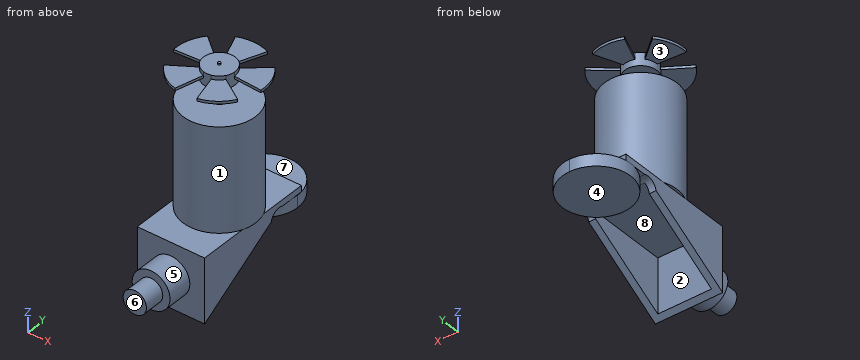
from build123d import *

# Parameters (mm, degrees)
F1_DEPTH  = 50.8
F2_R      = 3.175
F3_DEPTH  = 2.54
F4_R      = 0.635
F5_DEPTH  = 8.0518
F6_R      = 7.7597
F7_DEPTH  = 3.175
F9_DEPTH  = 1.27
F10_DEPTH = 3.175
F11_R     = 0.635
F12_DEPTH = 0.8382
F14_DEPTH = 31.496
F16_DEPTH = 51.816
F18_W     = 26.3473056257
F18_H     = 54.6325752512
F19_DEPTH = 28.448
F21_DEPTH = 5.9436
F22_R     = 9.271
F23_DEPTH = 12.3317
F26_R     = 5.715
F27_DEPTH = 10.16


# Not quite as in the source:
# - a length typed as a fraction of an inch, garbled in the dataset ("3 / 203.2 mm" for 3/8 in), is restored


with BuildPart() as f1:
    # F0 (on Top) → F1 (new body)
    with BuildSketch(Plane.XY):
        with BuildLine():
            Line((0, 35.56), (0, 0))
            ThreePointArc((0, 0), (12.5723585695, 5.2076414305), (17.78, 17.78))
            ThreePointArc((17.78, 17.78), (12.5723585695, 30.3523585695), (0, 35.56))
        make_face()
        with BuildLine():
            ThreePointArc((0, 35.56), (-17.78, 17.78), (0, 0))
            Line((0, 0), (0, 35.56))
        make_face()
    extrude(amount=F1_DEPTH)

    # F2 (on face) → F3 (join)
    with BuildSketch(Plane.XY.offset(50.8)):
        with Locations((0, 17.78)):
            Circle(F2_R)
    extrude(amount=F3_DEPTH)

    # F4 (on face) → F5 (join)
    with BuildSketch(Plane.XY.offset(53.34)):
        with Locations((0, 17.78)):
            Circle(F4_R)
    extrude(amount=F5_DEPTH)

    # F6 (on face) → F7 (join)
    with BuildSketch(Plane.XY.offset(61.3918)):
        with Locations((0, 17.78)):
            Circle(F6_R)
    extrude(amount=F7_DEPTH)

    # F8 (on face) → F9 (join)
    with BuildSketch(Plane.XY.offset(64.5668)):
        with BuildLine():
            Line((-7.8562656417, 37.7526283264), (-2.8404457135, 25.0011364922))
            ThreePointArc((-2.8404457135, 25.0011364922), (0, 25.4905939517), (2.8404457135, 25.0011364922))
            Line((2.8404457135, 25.0011364922), (7.8562656417, 37.7526283264))
            ThreePointArc((7.8562656417, 37.7526283264), (0, 39.3496460261), (-7.8562656417, 37.7526283264))
        make_face()
        with BuildLine():
            ThreePointArc((-7.745454913, 17.3100294897), (-7.3332106223, 20.1627045678), (-5.9899629188, 22.7128782998))
            Line((-5.9899629188, 22.7128782998), (-16.5673787218, 31.4236342075))
            ThreePointArc((-16.5673787218, 31.4236342075), (-20.5139524073, 24.4453871847), (-21.422817913, 16.4801289429))
            Line((-21.422817913, 16.4801289429), (-7.745454913, 17.3100294897))
        make_face()
        with BuildLine():
            ThreePointArc((-1.946508681, 10.2684057588), (-4.5321734112, 11.5419984564), (-6.5424463887, 13.6075499595))
            Line((-6.5424463887, 13.6075499595), (-18.0954687963, 6.2396013439))
            ThreePointArc((-18.0954687963, 6.2396013439), (-12.6783198313, 0.3297898022), (-5.3837639633, -2.9959928207))
            Line((-5.3837639633, -2.9959928207), (-1.946508681, 10.2684057588))
        make_face()
        with BuildLine():
            ThreePointArc((6.5424463887, 13.6075499595), (4.5321734112, 11.5419984564), (1.946508681, 10.2684057588))
            Line((1.946508681, 10.2684057588), (5.3837639633, -2.9959928207))
            ThreePointArc((5.3837639633, -2.9959928207), (12.6783198313, 0.3297898022), (18.0954687963, 6.2396013439))
            Line((18.0954687963, 6.2396013439), (6.5424463887, 13.6075499595))
        make_face()
        with BuildLine():
            ThreePointArc((5.9899629188, 22.7128782998), (7.3332106223, 20.1627045678), (7.745454913, 17.3100294897))
            Line((7.745454913, 17.3100294897), (21.422817913, 16.4801289429))
            ThreePointArc((21.422817913, 16.4801289429), (20.5139524073, 24.4453871847), (16.5673787218, 31.4236342075))
            Line((16.5673787218, 31.4236342075), (5.9899629188, 22.7128782998))
        make_face()
    extrude(amount=F9_DEPTH)

    # F10 (add): a face of the model
    f10_faces = [f1.faces().sort_by_distance(p)[0] for p in [
        (0, 17.78, 64.5668),
    ]]
    extrude(f10_faces, amount=F10_DEPTH)

    # F11 (on face) → F12 (join)
    with BuildSketch(Plane.XY.offset(67.7418)):
        with Locations((0, 17.78)):
            Circle(F11_R)
    extrude(amount=F12_DEPTH)

    # F13 (on face) → F14 (join)
    with BuildSketch(Plane(origin=(0, 0, 0), x_dir=(1, 0, 0), z_dir=(0, 0, -1))):
        with BuildLine():
            Line((-16.51, 12.319), (-16.51, -11.1808864232))
            ThreePointArc((-16.51, -11.1808864232), (0, 0), (16.51, -11.1808864232))
            Line((16.51, -11.1808864232), (16.51, 12.319))
            Line((16.51, 12.319), (-16.51, 12.319))
        make_face()
        with BuildLine():
            ThreePointArc((16.51, -24.3791135768), (0, -35.56), (-16.51, -24.3791135768))
            Line((-16.51, -24.3791135768), (-16.51, -47.879))
            Line((-16.51, -47.879), (16.51, -47.879))
            Line((16.51, -47.879), (16.51, -24.3791135768))
        make_face()
        with BuildLine():
            Line((-16.51, -11.1808864232), (-16.51, -17.78))
            Line((-16.51, -17.78), (-16.51, -24.3791135768))
            ThreePointArc((-16.51, -24.3791135768), (0, -35.56), (16.51, -24.3791135768))
            Line((16.51, -24.3791135768), (16.51, -17.78))
            Line((16.51, -17.78), (16.51, -11.1808864232))
            ThreePointArc((16.51, -11.1808864232), (0, 0), (-16.51, -11.1808864232))
        make_face()
    extrude(amount=F14_DEPTH)

    # F15 (on face) → F16 (cut)
    with BuildSketch(Plane.YZ.offset(16.51)):
        with BuildLine():
            Line((29.1356388479, -6.6541871056), (-12.319, -31.496))
            Line((-12.319, -31.496), (47.879, -31.496))
            Line((47.879, -31.496), (47.879, -3.048))
            Line((47.879, -3.048), (36.2268202007, -3.048))
            ThreePointArc((36.2268202007, -3.048), (31.8141050009, -3.1459858946), (29.1356388479, -6.6541871056))
        make_face()
    extrude(amount=-F16_DEPTH, mode=Mode.SUBTRACT)

    # F18 (on offset) → F19 (cut)
    with BuildSketch(Plane.XY.offset(-31.496)):
        with Locations((0, 17.7540327422)):
            Rectangle(F18_W, F18_H)
    extrude(amount=F19_DEPTH, mode=Mode.SUBTRACT)

    # F20 (on face) → F21 (join)
    with BuildSketch(Plane(origin=(0, 0, -3.048), x_dir=(1, 0, 0), z_dir=(0, 0, -1))):
        with BuildLine():
            ThreePointArc((0, -61.9528820528), (11.813335281, -57.0596383625), (16.7065789713, -45.2463030815))
            ThreePointArc((16.7065789713, -45.2463030815), (-11.813335281, -33.4329678005), (0, -61.9528820528))
        make_face()
    extrude(amount=F21_DEPTH)

    # F22 (on face) → F23 (join)
    with BuildSketch(Plane.XZ.offset(12.319)):
        with Locations((0, -15.748)):
            Circle(F22_R)
    extrude(amount=F23_DEPTH)

    # F26 (on face) → F27 (join)
    with BuildSketch(Plane.XZ.offset(24.6507)):
        with Locations((0, -15.748)):
            Circle(F26_R)
    extrude(amount=F27_DEPTH)


solid = f1.part
Here's how the part is built. I have some questions about the finished solid (model axes, mm). Face numbers are marked on the shaded views. A direction names the side the tool comes from. Give positions to 0.01 mm unless a question says otherwise; leave off trailing zeros. Write each loop counter-clockwise with the first axis right and the second up, starting at its lowest first coordinate (ties: lowest second). Pieces come first, ordered by that corner, then holes. Notation, with made-up numbers: (86, 57) -> (94, 57) arc R14 cw to (94, 64) -> close; hole circle Ø10 at (87, -17). An arc over 180 degrees is marked (long way). Use one line per item in the form item = value. Start each with the question number.
1. Will these pins go through, and if not, where does the flat tip stop? pin 1 Ø4 at (x, y) = (5, 44.5) entering from +Z; pin 2 Ø7.5 at (x, y) = (13.5, 22.5) entering from +Z; pin 3 Ø3 at (x, z) = (-14.5, 26) entering from +Y; pin 4 Ø7.5 at (x, y) = (0, 20) entering from +Z.
2. On a 3-axis mill with a long thin cutter (end or side, diameter ignored), from which of +Z, -Z, +X, -X, +Y, -Y can I reach the whole of each face in a straight line? I mean the marked faces 4, 5, 6, 7 and 8. Say none if no direction works.
3. Imagine slicing it at B-B on y = 50. List the corners of the cut face in (x, z) for me, plus the area to 3 significant figures.
4. Thinking about a two-plate mould opening in X: for the marked faces 1, 2 and 3, which applies, +X half, -X half, draft (parallel to the pull), parting line (faces both ways), or undercut?
5. If I drill on L1, parallel to X at y = -5.5, z = -23; L2, parallel to Z at x = 4, y = 2.5; L3, parallel to Z at x = 6, y = 23, over which ranges is the centre line in solid material (lowest first)?
6. Imagine slicing it at A-A on z = 32.5. List the corners of the cut face in (x, y) for me.
Entries:
q1.pin_1 = 0
q1.pin_2 = 65.84
q1.pin_3 = 29.91
q1.pin_4 = 68.58
q2.face_4 = -Z, +X, -X, +Y
q2.face_5 = -Y
q2.face_6 = +Z, -Z, +X, -X, -Y
q2.face_7 = +Z, +X, -X, +Y
q2.face_8 = -Z
q3.outline = (-16.02, -8.99) -> (16.02, -8.99) -> (16.02, -3.05) -> (-16.02, -3.05) -> close
q3.area = 190 mm²
q4.face_1 = parting line
q4.face_2 = undercut
q4.face_3 = draft
q5.L1 = -16.51 to -13.17, 13.17 to 16.51
q5.L2 = -3.05 to 50.8, 64.57 to 65.84
q5.L3 = -3.05 to 50.8
q6.outline = circle Ø35.56 at (0, 17.78)
